The model under review builds one solid part; all positions refer to its coordinate system, in mm. A direction names the side the tool comes from. Give positions to 0.01 mm unless a question says otherwise; leave off trailing zeros. Write each loop counter-clockwise with the first axis right and the second up, starting at its lowest first coordinate (ties: lowest second). Pieces come first, ordered by that corner, then holes. Notation, with made-up numbers: M 32,4 L 89,4 A11 ccw 89,22 Z; hole C -31.75,-30.5 d10. An arc over 180 degrees is marked long. Write each question's results on one line, items separated by ' | '. Start each with the question number.
from build123d import *

# Parameters (mm, degrees)
CROQUIS1_R                    = 8
SALIENTE_EXTRUIR1_DEPTH       = 10
CROQUIS2_R                    = 7
CORTAR_EXTRUIR1_DEPTH         = 8
CROQUIS3_R                    = 5
SALIENTE_EXTRUIR2_DEPTH       = 14
CROQUIS4_R                    = 3.5
CORTAR_EXTRUIR2_DEPTH         = 14
CROQUIS5_W                    = 8.830556774
CROQUIS5_H                    = 0.810001326
SALIENTE_EXTRUIR3_DEPTH       = 14
SALIENTE_EXTRUIR4_START       = -10
SALIENTE_EXTRUIR4_OUTLINE_R   = 7
SALIENTE_EXTRUIR4_OUTLINE_R_2 = 6.177042676
SALIENTE_EXTRUIR4_DEPTH       = 8
CORTAR_EXTRUIR10_DEPTH        = 10
SALIENTE_EXTRUIR7_START       = -14
CROQUIS12_R                   = 3.5
CROQUIS12_R_2                 = 3.1
SALIENTE_EXTRUIR7_DEPTH       = 14
CROQUIS14_R                   = 5.293122991
CROQUIS14_R_2                 = 4.002052416
CORTAR_EXTRUIR15_DEPTH        = 14


# Read off the part's stored shape, not the designer's step: Saliente-Extruir4
with BuildPart() as part:
    # Croquis1 → Saliente-Extruir1 (new body)
    with BuildSketch(Plane.XY):
        Circle(CROQUIS1_R)
    extrude(amount=SALIENTE_EXTRUIR1_DEPTH)

    # Croquis2 → Cortar-Extruir1 (cut)
    with BuildSketch(Plane.XY.offset(10)):
        Circle(CROQUIS2_R)
    extrude(amount=-CORTAR_EXTRUIR1_DEPTH, mode=Mode.SUBTRACT)

    # Croquis3 → Saliente-Extruir2 (add)
    with BuildSketch(Plane.XY.offset(2)):
        Circle(CROQUIS3_R)
    extrude(amount=SALIENTE_EXTRUIR2_DEPTH)

    # Croquis4 → Cortar-Extruir2 (cut)
    with BuildSketch(Plane.XY.offset(16)):
        Circle(CROQUIS4_R)
    extrude(amount=-CORTAR_EXTRUIR2_DEPTH, mode=Mode.SUBTRACT)

    # Croquis5 → Saliente-Extruir3 (add)
    with BuildSketch(Plane.XY.offset(2)):
        Rectangle(CROQUIS5_W, CROQUIS5_H)
    extrude(amount=SALIENTE_EXTRUIR3_DEPTH)

    # Saliente-Extruir4 outline → Saliente-Extruir4 (add)
    with BuildSketch(Plane(origin=(0, 0, 0), x_dir=(-1, 0, 0), z_dir=(0, 0, -1)).offset(SALIENTE_EXTRUIR4_START)):
        Circle(SALIENTE_EXTRUIR4_OUTLINE_R)
        Circle(SALIENTE_EXTRUIR4_OUTLINE_R_2, mode=Mode.SUBTRACT)
    extrude(amount=SALIENTE_EXTRUIR4_DEPTH)

    # Croquis11 → Cortar-Extruir10 (cut)
    with BuildSketch(Plane(origin=(0, 0, 0), x_dir=(-1, 0, 0), z_dir=(0, 0, -1))):
        with BuildLine():
            Line((-0.247260298, 7.379594776), (-0.5002941, 8.108053777))
            Line((-0.5002941, 8.108053777), (1.061510951, 8.036738478))
            Line((1.061510951, 8.036738478), (0.736778233, 7.346884683))
            ThreePointArc((0.736778233, 7.346884683), (0.245304789, 7.379660038), (-0.247260298, 7.379594776))
        make_face()
        with BuildLine():
            Line((2.029718445, 7.865816758), (3.493045676, 7.315367575))
            Line((3.493045676, 7.315367575), (2.971029962, 6.759625557))
            ThreePointArc((2.971029962, 6.759625557), (2.513739083, 6.942670418), (2.045261679, 7.094819334))
            Line((2.045261679, 7.094819334), (2.029718445, 7.865816758))
        make_face()
        with BuildLine():
            Line((4.137579194, 6.115553542), (4.361048006, 6.853618791))
            Line((4.361048006, 6.853618791), (5.582656753, 5.877917526))
            Line((5.582656753, 5.877917526), (4.914456579, 5.510687185))
            ThreePointArc((4.914456579, 5.510687185), (4.536111081, 5.826083846), (4.137579194, 6.115553542))
        make_face()
        with BuildLine():
            Line((5.824881629, 4.537654761), (6.265487803, 5.170540864))
            Line((6.265487803, 5.170540864), (7.12579849, 3.865095955))
            Line((7.12579849, 3.865095955), (6.376821944, 3.722324356))
            ThreePointArc((6.376821944, 3.722324356), (6.114456921, 4.139199594), (5.824881629, 4.537654761))
        make_face()
        with BuildLine():
            Line((6.942004065, 2.515578715), (7.556618, 2.981334372))
            Line((7.556618, 2.981334372), (7.971417423, 1.473931862))
            Line((7.971417423, 1.473931862), (7.214979548, 1.569594483))
            ThreePointArc((7.214979548, 1.569594483), (7.094277116, 2.047141646), (6.942004065, 2.515578715))
        make_face()
        with BuildLine():
            Line((7.379594776, 0.247260298), (8.108053777, 0.5002941))
            Line((8.108053777, 0.5002941), (8.036738478, -1.061510951))
            Line((8.036738478, -1.061510951), (7.346884683, -0.736778233))
            ThreePointArc((7.346884683, -0.736778233), (7.379660038, -0.245304789), (7.379594776, 0.247260298))
        make_face()
        with BuildLine():
            Line((7.094819334, -2.045261679), (7.865816758, -2.029718445))
            Line((7.865816758, -2.029718445), (7.315367575, -3.493045676))
            Line((7.315367575, -3.493045676), (6.759625557, -2.971029962))
            ThreePointArc((6.759625557, -2.971029962), (6.942670418, -2.513739083), (7.094819334, -2.045261679))
        make_face()
        with BuildLine():
            Line((6.115553542, -4.137579194), (6.853618791, -4.361048006))
            Line((6.853618791, -4.361048006), (5.877917526, -5.582656753))
            Line((5.877917526, -5.582656753), (5.510687185, -4.914456579))
            ThreePointArc((5.510687185, -4.914456579), (5.826083846, -4.536111081), (6.115553542, -4.137579194))
        make_face()
        with BuildLine():
            Line((4.537654761, -5.824881629), (5.170540864, -6.265487803))
            Line((5.170540864, -6.265487803), (3.865095955, -7.12579849))
            Line((3.865095955, -7.12579849), (3.722324356, -6.376821944))
            ThreePointArc((3.722324356, -6.376821944), (4.139199594, -6.114456921), (4.537654761, -5.824881629))
        make_face()
        with BuildLine():
            Line((2.515578715, -6.942004065), (2.981334372, -7.556618))
            Line((2.981334372, -7.556618), (1.473931862, -7.971417423))
            Line((1.473931862, -7.971417423), (1.569594483, -7.214979548))
            ThreePointArc((1.569594483, -7.214979548), (2.047141646, -7.094277116), (2.515578715, -6.942004065))
        make_face()
        with BuildLine():
            Line((0.247260298, -7.379594776), (0.5002941, -8.108053777))
            Line((0.5002941, -8.108053777), (-1.061510951, -8.036738478))
            Line((-1.061510951, -8.036738478), (-0.736778233, -7.346884683))
            ThreePointArc((-0.736778233, -7.346884683), (-0.245304789, -7.379660038), (0.247260298, -7.379594776))
        make_face()
        with BuildLine():
            Line((-2.045261679, -7.094819334), (-2.029718445, -7.865816758))
            Line((-2.029718445, -7.865816758), (-3.493045676, -7.315367575))
            Line((-3.493045676, -7.315367575), (-2.971029962, -6.759625557))
            ThreePointArc((-2.971029962, -6.759625557), (-2.513739083, -6.942670418), (-2.045261679, -7.094819334))
        make_face()
        with BuildLine():
            Line((-4.137579194, -6.115553542), (-4.361048006, -6.853618791))
            Line((-4.361048006, -6.853618791), (-5.582656753, -5.877917526))
            Line((-5.582656753, -5.877917526), (-4.914456579, -5.510687185))
            ThreePointArc((-4.914456579, -5.510687185), (-4.536111081, -5.826083846), (-4.137579194, -6.115553542))
        make_face()
        with BuildLine():
            Line((-5.824881629, -4.537654761), (-6.265487803, -5.170540864))
            Line((-6.265487803, -5.170540864), (-7.12579849, -3.865095955))
            Line((-7.12579849, -3.865095955), (-6.376821944, -3.722324356))
            ThreePointArc((-6.376821944, -3.722324356), (-6.114456921, -4.139199594), (-5.824881629, -4.537654761))
        make_face()
        with BuildLine():
            Line((-6.942004065, -2.515578715), (-7.556618, -2.981334372))
            Line((-7.556618, -2.981334372), (-7.971417423, -1.473931862))
            Line((-7.971417423, -1.473931862), (-7.214979548, -1.569594483))
            ThreePointArc((-7.214979548, -1.569594483), (-7.094277116, -2.047141646), (-6.942004065, -2.515578715))
        make_face()
        with BuildLine():
            Line((-7.379594776, -0.247260298), (-8.108053777, -0.5002941))
            Line((-8.108053777, -0.5002941), (-8.036738478, 1.061510951))
            Line((-8.036738478, 1.061510951), (-7.346884683, 0.736778233))
            ThreePointArc((-7.346884683, 0.736778233), (-7.379660038, 0.245304789), (-7.379594776, -0.247260298))
        make_face()
        with BuildLine():
            Line((-7.094819334, 2.045261679), (-7.865816758, 2.029718445))
            Line((-7.865816758, 2.029718445), (-7.315367575, 3.493045676))
            Line((-7.315367575, 3.493045676), (-6.759625557, 2.971029962))
            ThreePointArc((-6.759625557, 2.971029962), (-6.942670418, 2.513739083), (-7.094819334, 2.045261679))
        make_face()
        with BuildLine():
            Line((-6.115553542, 4.137579194), (-6.853618791, 4.361048006))
            Line((-6.853618791, 4.361048006), (-5.877917526, 5.582656753))
            Line((-5.877917526, 5.582656753), (-5.510687185, 4.914456579))
            ThreePointArc((-5.510687185, 4.914456579), (-5.826083846, 4.536111081), (-6.115553542, 4.137579194))
        make_face()
        with BuildLine():
            Line((-4.537654761, 5.824881629), (-5.170540864, 6.265487803))
            Line((-5.170540864, 6.265487803), (-3.865095955, 7.12579849))
            Line((-3.865095955, 7.12579849), (-3.722324356, 6.376821944))
            ThreePointArc((-3.722324356, 6.376821944), (-4.139199594, 6.114456921), (-4.537654761, 5.824881629))
        make_face()
        with BuildLine():
            Line((-2.515578715, 6.942004065), (-2.981334372, 7.556618))
            Line((-2.981334372, 7.556618), (-1.473931862, 7.971417423))
            Line((-1.473931862, 7.971417423), (-1.569594483, 7.214979548))
            ThreePointArc((-1.569594483, 7.214979548), (-2.047141646, 7.094277116), (-2.515578715, 6.942004065))
        make_face()
    extrude(amount=-CORTAR_EXTRUIR10_DEPTH, mode=Mode.SUBTRACT)

    # Croquis12 → Saliente-Extruir7 (add)
    with BuildSketch(Plane.XY.offset(16).offset(SALIENTE_EXTRUIR7_START)):
        Circle(CROQUIS12_R)
        Circle(CROQUIS12_R_2, mode=Mode.SUBTRACT)
    extrude(amount=SALIENTE_EXTRUIR7_DEPTH)

    # Croquis14 → Cortar-Extruir15 (cut)
    with BuildSketch(Plane.XY.offset(16)):
        Circle(CROQUIS14_R)
        Circle(CROQUIS14_R_2, mode=Mode.SUBTRACT)
    extrude(amount=-CORTAR_EXTRUIR15_DEPTH, mode=Mode.SUBTRACT)


solid = part.part
(1) Add section C-C (x = 0). State the section outline as (y, z) points (3 decimals), then the cut area to 3 significant figures.
(2) Machinability: for faces 4 (the cylindrical face through (0.98, 7.94, 4.93)), 5 (the cylindrical face through (-7.38, -0.25, 4.93)), 6 (the flat face through (0, -1, 2)), 7 (the cylindrical face through (6.94, 2.52, 4.93)), 8 (the cylindrical face through (-0.98, -7.94, 4.93)), which of the approach directions +Z, -Z, +X, -X, +Y, -Y give a long, thin tool a straight path to every point of the face, cutting with its end or side? Answer none if there is none.
(3) Clearance check with flat-ended pins moving along their axes: P1, Ø6, axis at y = -6, z = 6, coming from the -X side; P2, Ø1.8, axis at x = 0.5, z = 8.5, coming from the -Y side; P3, Ø2, axis at x = 2.5, z = 11.5, coming from the -Y side. State where each tip first meets the part, or that it passes through.
(4) Add section A-A (z = 4.75). Give the number of separate pieces and of enclosed holes in the cut face, then the cut area to 3 significant figures.
(5) Draft analysis for pull direction X (two halves, no side actions). For faces 1 (the cylindrical face through (7.854, 1.519, 4.93)), 2 (the cylindrical face through (-4.13, -6.12, 4.93)), 3 (the cylindrical face through (-7.096, 2.041, 4.93)), state which applies: pulls with the +X half, pulls with the -X half, needs draft (parallel to the pull), parting line crosses it, or undercut.
(6) Add section D-D (z = 10.25). State the section outline as (x, y) points (3 decimals).
(7) Wall thickness on L1, parallel to Y at x = 1.25, z = 14.5 (3 decimals); L2, parallel to X at y = 2.25, z = 2.5; L3, parallel to Z at x = 1.25, y = -2.5: over which ranges is each line inside the solid? List them lowest first.
(8) Add section B-B (y = 0). State the section outline as (x, z) points.
Calculated:
1) outline: M -7.384,0 L 7.384,0 L 7.384,10 L 6.177,10 L 6.177,2 L 4.002,2 L 4.002,16 L 3.1,16 L 3.1,2 L 0.405,2 L 0.405,16 L -0.405,16 L -0.405,2 L -3.1,2 L -3.1,16 L -4.002,16 L -4.002,2 L -6.177,2 L -6.177,10 L -7.384,10 Z | area: 85.4 mm²
2) face 4: +Z, -Z, +X, +Y | face 5: +Z, -Z, -X | face 6: +Z | face 7: +Z, -Z, +X | face 8: +Z, -Z, -X, -Y
3) P1: stops at x = -7.23 | P2: stops at y = -7.94 | P3: stops at y = -3.71
4) separate pieces: 2 | enclosed holes: 3 | area: 91.2 mm²
5) face 1: pulls with the +X half | face 2: undercut | face 3: pulls with the -X half
6) outline: C 0,0 d8.004; hole M -3.073,-0.405 A3.1 ccw 3.073,-0.405 Z; hole M -3.073,0.405 L 3.073,0.405 A3.1 ccw Z
7) L1: y = -3.802 to -2.837, -0.405 to 0.405, 2.837 to 3.802 | L2: x = -7.03 to -5.75, -3.31 to -2.13, 2.13 to 3.31, 5.75 to 7.03 | L3: z = 0 to 2
8) outline: M -7.38,0 L 7.38,0 L 7.38,10 L 6.18,10 L 6.18,2 L 4,2 L 4,16 L -4,16 L -4,2 L -6.18,2 L -6.18,10 L -7.38,10 Z
